Autodesk Inventor part; units mm, degrees
ref_plane "YZ Plane" through (0, 0, 0) normal (1, 0, 0) x (0, 1, 0)
ref_plane "XZ Plane" through (0, 0, 0) normal (0, 1, 0) x (-1, 0, 0)
ref_plane "XY Plane" through (0, 0, 0) normal (0, 0, 1) x (1, 0, 0)
sketch "Sketch1" plane through (0, 0, 0) normal (0, 0, 1) x (1, 0, 0)
  line L0 (0, 0) -> (400, 0)
  line L1 (400, 0) -> (400, 350)
  line L2 (400, 350) -> (0, 350)
  line L3 (0, 350) -> (0, 0)
  dimension "d0" = 400
  dimension "d1" = 350
extrude "Extrusion1" add sketch "Sketch1" along normal blind 20
sketch "Sketch7" plane through (0, 0, 20) normal (0, 0, 1) x (1, 0, 0)
  circle A0 centre (40, 40) radius 5.053
  line L0 (400, 350) -> (0, 350) construction
  line L1 (400, 0) -> (400, 350) construction
  line L2 (0, 0) -> (400, 0) construction
  line L3 (0, 350) -> (0, 0) construction
  line L4 (200, 350) -> (200, 0) construction
  line L5 (0, 175) -> (400, 175) construction
  circle A1 centre (40, 310) radius 5.053
  circle A2 centre (360, 40) radius 5.053
  circle A3 centre (360, 310) radius 5.053
extrude "Extrusion7" cut sketch "Sketch7" against normal blind 20
sketch "Sketch8" plane through (0, 0, 0) normal (0, 0, -1) x (-1, 0, 0)
  circle A0 centre (-309.525, 175) radius 3
  circle A1 centre (-328.575, 175) radius 3
  point P0 (0, 0)
extrude "Extrusion8" cut sketch "Sketch8" against normal blind 20
sketch "Sketch9" plane through (0, 0, 0) normal (0, 0, -1) x (-1, 0, 0)
  circle A0 centre (-309.525, 175) radius 3 construction
  circle A1 centre (-328.575, 175) radius 3 construction
  circle A2 centre (-309.525, 175) radius 3
  circle A3 centre (-309.525, 175) radius 5
  circle A4 centre (-328.575, 175) radius 3
  circle A5 centre (-328.575, 175) radius 5
  point P0 (0, 0)
  dimension "d24" = 10
  dimension "d25" = 10
extrude "Extrusion9" cut sketch "Sketch9" against normal blind 6
equation "\"d0\" = maxl"
equation "\"d1\" = maxw"
equation "\"d2\" = platft"
equation "\"d20\" = platft"
equation "\"d22\" = platft"
equation "\"d24\" = bhd"
equation "\"d25\" = bhd"
equation "\"d26\" = bhh"
equation "\"dias\" = 8.8"
equation "\"stra1\" = 9.5"
equation "\"diab2\" = 6"
equation "\"stra\" = 25"
equation "\"db1\" = 6"
equation "\"ds1\" = 5.8"
equation "\"ds2\" = 1.6"
equation "\"ang\" = 120deg"
equation "\"db2\" = 3"
equation "\"diab3\" = 7"
equation "\"diab4\" = 3"
equation "\"dias1\" = 13.4375"
equation "\"dias3\" = 2"
equation "\"dias4\" = 4"
equation "\"t1\" = 3"
equation "\"t2\" = 3"
equation "\"t3\" = 6"
equation "\"t4\" = 6"
equation "\"t5\" = 3"
equation "\"diab1\" = 19"
equation "\"afw\" = 0.2"
equation "\"maxw\" = 350"
equation "\"lcsd\" = 19.05"
equation "\"lcwd1\" = 25"
equation "\"lch1\" = 39"
equation "\"lcwd2\" = 34"
equation "\"lcwd3\" = 43"
equation "\"dia1\" = 6"
equation "\"td\" = 18"
equation "\"bhh\" = 6"
equation "\"bhd\" = 10"
equation "\"spacert\" = 2"
equation "\"sw\" = 25"
equation "\"sh\" = 31"
equation "\"platft\" = 20"
equation "\"pvct\" = 5"
equation "\"tankl\" = 379"
equation "\"dia4\" = 11"
equation "\"dia3\" = 8"
equation "\"play\" = 9"
equation "\"holeh\" = 26"
equation "\"surroundt\" = 5"
equation "\"slack\" = 0.5"
equation "\"play2\" = 3"
equation "\"maxl\" = 400"
equation "\"diaoverflow\" = 25"
equation "\"diacucl\" = 32"
equation "\"diawater\" = 25"
equation "\"diaph\" = 32"
equation "\"diaair\" = 32"
equation "\"diasurroundhole\" = 42"
equation "\"diagrate\" = 12"
equation "\"gratespacing\" = 12.02082"
equation "\"sidedist\" = 13.9375"
equation "\"bottomdist\" = 9.6355"
equation "\"diahcl\" = 32"
equation "\"bracketwtop\" = 6"
equation "\"bracketwbottom\" = 6"
equation "\"nett\" = 1"
equation "\"nethole\" = 16"
equation "\"nettop\" = 7"
equation "\"netside\" = 3.5"
equation "\"netholespacing\" = 2"
equation "\"diaetape\" = 32"
properties part number "platform_top" material "PVC-Piping"
Part model, mm, in its own coordinate system. A direction names the side the tool comes from. Give positions to 0.01 mm unless a question says otherwise; leave off trailing zeros. Loops run counter-clockwise (first coordinate to the right, second up) from the corner with the lowest first, then second, coordinate; pieces in that order, holes last.
(1) Drill centre lines: line 1 along Y through (x, z) = (360, 8.25); line 2 along X through (y, z) = (176, 13.5); line 3 along X through (y, z) = (308.5, 19). Where is each one in solid material? Low to high.
Return value:
line 1: y = 0 to 34.95, 45.05 to 304.95, 315.05 to 350
line 2: x = 0 to 306.7, 312.35 to 325.75, 331.4 to 400
line 3: x = 0 to 35.17, 44.83 to 355.17, 364.83 to 400
(2) Pull direction Y, two halves, no side cores. Call faces 3 (the flat face through (400, 173, 10)), 4 (the flat face through (307, 173, 6)), 5 (the flat face through (197, 0, 10)), 6 (the cylindrical face through (333.57, 175.22, 2.96)): pulls with the +Y half, pulls with the -Y half, needs draft (parallel to the pull), parting line crosses it, or undercut.
Return value:
face 3: needs draft
face 4: undercut
face 5: pulls with the -Y half
face 6: undercut
(3) 3-axis set-ups, long thin cutter, end or side, ignore diameter. For faces 1 (the flat face through (0, 177, 10)), 2 (the cylindrical face through (304.756, 176.502, 2.958)): which of +Z, -Z, +X, -X, +Y, -Y reach the whole face in a straight line?
Return value:
face 1: +Z, -Z, -X, +Y, -Y
face 2: -Z
(4) Band-saw the part on A-A (y = 40). Write the cut outline in (x, z).
Return value:
outline: (0, 0) - (34.95, 0) - (34.95, 20) - (0, 20) - close; (45.05, 0) - (354.95, 0) - (354.95, 20) - (45.05, 20) - close; (365.05, 0) - (400, 0) - (400, 20) - (365.05, 20) - close
(5) Pin check, flat tips, straight feed: pin 1 (10 mm diameter, centred on y = 121, z = 5.5, fed in from -X); pin 2 (8 mm diameter, centred on x = 40, y = 40, fed in from +Z). Stop position of each tip, or through.
Return value:
pin 1: stops at x = 0
pin 2: passes through
(6) Band-saw the part on B-B (x = 360). Write the cut outline in (y, z).
Return value:
outline: (0, 0) - (34.95, 0) - (34.95, 20) - (0, 20) - close; (45.05, 0) - (304.95, 0) - (304.95, 20) - (45.05, 20) - close; (315.05, 0) - (350, 0) - (350, 20) - (315.05, 20) - close
